```python
from build123d import *
from build123d.topology import SkipClean

# Parameters (mm, degrees)
SKETCH_1_W          = 20
SKETCH_1_H          = 12
SKETCH_1_R          = 2.05
SKETCH_1_R_2        = 3.5
EXTRUDE_1_DEPTH     = 2
CUT_EXTRUDE_START   = 2
SKETCH_1_3_R        = 1.6
CUT_EXTRUDE_6_DEPTH = 1
SKETCH_3_W          = 20
SKETCH_3_H          = 12
EXTRUDE_3_DEPTH     = 1.4
EXTRUDE_START       = 1.4
SKETCH_3_17_W       = 20
SKETCH_3_17_H       = 12
EXTRUDE_4_DEPTH     = 1.7
CUT_EXTRUDE_START_2 = 5.1
SKETCH_5_R          = 0.9
CUT_EXTRUDE_1_DEPTH = 29.974882199
SKETCH_5_10_R       = 1.5
CUT_EXTRUDE_3_DEPTH = 4.6
SKETCH_7_R          = 0.35
SKETCH_7_R_2        = 0.7
CUT_EXTRUDE_4_DEPTH = 24.874882199
SKETCH_7_3_R        = 1
CUT_EXTRUDE_7_DEPTH = 3.1


with BuildPart() as part:
    # 草图1 → 凸台-拉伸1 (new body)
    with BuildSketch(Plane(origin=(0, 0, 0), x_dir=(1, 0, 0), z_dir=(0, 1, 0))):
        with Locations((10, -6)):
            Rectangle(SKETCH_1_W, SKETCH_1_H)
        with Locations(Location((5, -6, 0), (0, 0, 270))):
            Circle(SKETCH_1_R, mode=Mode.SUBTRACT)
        with Locations(Location((15, -6, 0), (0, 0, 270))):
            Circle(SKETCH_1_R_2, mode=Mode.SUBTRACT)
    extrude(amount=EXTRUDE_1_DEPTH)

    # 草图1<3> → 切除-拉伸6 (cut)
    with BuildSketch(Plane(origin=(0, 0, 0), x_dir=(1, 0, 0), z_dir=(0, 1, 0)).offset(CUT_EXTRUDE_START)):
        with Locations(Location((9.2, -6, 0), (0, 0, 270))):
            Circle(SKETCH_1_3_R)
    extrude(amount=-CUT_EXTRUDE_6_DEPTH, mode=Mode.SUBTRACT)

    # 草图3 → 凸台-拉伸3 (add)
    with SkipClean():  # the faces are left unmerged after this step: merging them gives an invalid solid
        with BuildSketch(Plane(origin=(0, 2, 0), x_dir=(1, 0, 0), z_dir=(0, 1, 0))):
            with Locations((10, -6)):
                Rectangle(SKETCH_3_W, SKETCH_3_H)
            with BuildLine():
                ThreePointArc((6.141964286, -7.702473956), (2.95, -6), (6.141964286, -4.297526044))
                ThreePointArc((6.141964286, -4.297526044), (9.04909865, -2.503254544), (12.1, -4.040408206))
                ThreePointArc((12.1, -4.040408206), (18.5, -6), (12.1, -7.959591794))
                ThreePointArc((12.1, -7.959591794), (9.04909865, -9.496745456), (6.141964286, -7.702473956))
            make_face(mode=Mode.SUBTRACT)
        extrude(amount=EXTRUDE_3_DEPTH)

    # 草图3<17> → 凸台-拉伸4 (add)
    with SkipClean():  # the faces are left unmerged after this step: merging them gives an invalid solid
        with BuildSketch(Plane(origin=(0, 2, 0), x_dir=(1, 0, 0), z_dir=(0, 1, 0)).offset(EXTRUDE_START)):
            with Locations((10, -6)):
                Rectangle(SKETCH_3_17_W, SKETCH_3_17_H)
            with BuildLine():
                ThreePointArc((6.141964286, -7.702473956), (2.95, -6), (6.141964286, -4.297526044))
                ThreePointArc((6.141964286, -4.297526044), (8.789071626, -2.524206872), (11.776724138, -3.631352133))
                ThreePointArc((11.776724138, -3.631352133), (16.246374051, -2.199138029), (19, -6))
                ThreePointArc((19, -6), (16.246374051, -9.800861971), (11.776724138, -8.368647867))
                ThreePointArc((11.776724138, -8.368647867), (8.789071626, -9.475793128), (6.141964286, -7.702473956))
            make_face(mode=Mode.SUBTRACT)
        extrude(amount=EXTRUDE_4_DEPTH)

    # 草图5 → 切除-拉伸1 (cut, through all)
    with SkipClean():  # the faces are left unmerged after this step: merging them gives an invalid solid
        with BuildSketch(Plane(origin=(0, 0, 0), x_dir=(1, 0, 0), z_dir=(0, 1, 0)).offset(CUT_EXTRUDE_START_2)):
            with Locations(Location((2.3, -2.214171161, 0), (0, 0, 270))):
                Circle(SKETCH_5_R)
            with Locations(Location((7.7, -9.785828839, 0), (0, 0, 270))):
                Circle(SKETCH_5_R)
        extrude(amount=-CUT_EXTRUDE_1_DEPTH, mode=Mode.SUBTRACT)

    # 草图5<10> → 切除-拉伸3 (cut)
    with SkipClean():  # the faces are left unmerged after this step: merging them gives an invalid solid
        with BuildSketch(Plane(origin=(0, 0, 0), x_dir=(1, 0, 0), z_dir=(0, 1, 0)).offset(CUT_EXTRUDE_START_2)):
            with Locations(Location((2.3, -2.214171161, 0), (0, 0, 270))):
                Circle(SKETCH_5_10_R)
            with Locations(Location((7.7, -9.785828839, 0), (0, 0, 270))):
                Circle(SKETCH_5_10_R)
        extrude(amount=-CUT_EXTRUDE_3_DEPTH, mode=Mode.SUBTRACT)

    # 草图7 → 切除-拉伸4 (cut, through all)
    with SkipClean():  # the faces are left unmerged after this step: merging them gives an invalid solid
        with BuildSketch(Plane(origin=(0, 5.1, 0), x_dir=(1, 0, 0), z_dir=(0, 1, 0))):
            with Locations(Location((6, -2, 0), (0, 0, 270))):
                Circle(SKETCH_7_R)
            with Locations(Location((3, -9, 0), (0, 0, 270))):
                Circle(SKETCH_7_R)
            with Locations(Location((17, -1.5, 0), (0, 0, 270))):
                Circle(SKETCH_7_R)
            with Locations(Location((17, -10.5, 0), (0, 0, 270))):
                Circle(SKETCH_7_R)
            with Locations(Location((11.5, -1.5, 0), (0, 0, 270))):
                Circle(SKETCH_7_R_2)
            with Locations(Location((18.5, -10.5, 0), (0, 0, 270))):
                Circle(SKETCH_7_R_2)
            with Locations(Location((11.5, -10.5, 0), (0, 0, 270))):
                Circle(SKETCH_7_R_2)
            with Locations(Location((18.5, -1.5, 0), (0, 0, 270))):
                Circle(SKETCH_7_R_2)
        extrude(amount=-CUT_EXTRUDE_4_DEPTH, mode=Mode.SUBTRACT)

    # 草图7<3> → 切除-拉伸7 (cut)
    with SkipClean():  # the faces are left unmerged after this step: merging them gives an invalid solid
        with BuildSketch(Plane(origin=(0, 5.1, 0), x_dir=(1, 0, 0), z_dir=(0, 1, 0))):
            with Locations(Location((11.5, -1.5, 0), (0, 0, 270))):
                Circle(SKETCH_7_3_R)
            with Locations(Location((18.5, -10.5, 0), (0, 0, 270))):
                Circle(SKETCH_7_3_R)
            with Locations(Location((11.5, -10.5, 0), (0, 0, 270))):
                Circle(SKETCH_7_3_R)
            with Locations(Location((18.5, -1.5, 0), (0, 0, 270))):
                Circle(SKETCH_7_3_R)
        extrude(amount=-CUT_EXTRUDE_7_DEPTH, mode=Mode.SUBTRACT)


solid = part.part
```
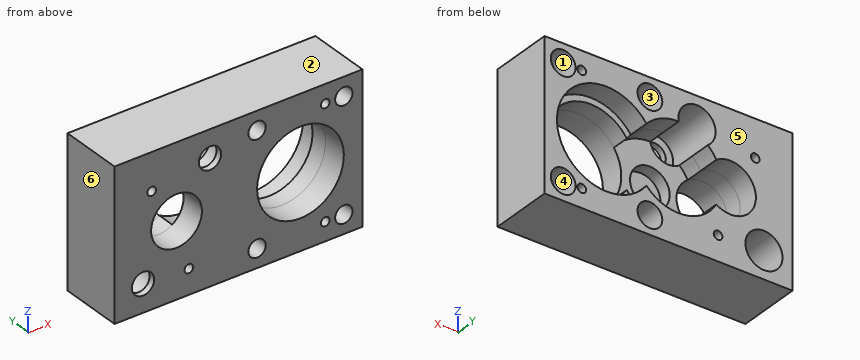
Work out the finished part from the listing and answer in its coordinate system (mm). Face numbers are marked on the shaded views. A direction names the side the tool comes from. Give positions to 0.01 mm unless a question says otherwise; leave off trailing zeros. Order: outer loops, then holes, each group sorted by start corner. A loop starts at its lowest first (then second) coordinate and runs counter-clockwise, first axis right, second up. Notation, with made-up numbers: (-30, -39) - (8, -39) arc R33 cw to (8, -4) - close; hole circle Ø4 at (35, 76.5). An arc over 180 degrees is marked (long way). One line per item, written item: value. Start each with the question number.
1. Section C-C, the plane y = 2.7 is taken. Count the separate pieces of the cut face and the enclosed holes in it, then the cut area to 3 significant figures.
2. Section D-D, the plane x = 5 is taken. Write down the section's boundary in (y, z), then the cut area to 3 significant figures.
3. Consider line 1 (Z direction, x = 2.75, y = 2.2); line 2 (X direction, y = 1.75, z = 5.25); line 3 (X direction, y = 3.05, z = 1.5). Determine where each line is inside the solid, lowest interval first.
4. Section A-A, the plane x = 15 is taken. Write down the section's boundary in (y, z), then the cut area to 3 significant figures.
5. Which of the six approach directions +Z, -Z, +X, -X, +Y, -Y give full straight-line access (tool end or side, diameter ignored) to the marked faces 1 and 2?
6. For a pull along X with two mould halves and no side action, classify the marked faces 3, 4, 5 and 6 as released by +X, released by -X, zero draft, split by the parting line, or undercut.
7. Each of these flat-tipped pins is pushed along its axis until it touches: pin 1 Ø2.5 at (x, z) = (18.5, 10.5) entering from -Y; pin 2 Ø1 at (x, z) = (18.5, 10.5) entering from +Y; pin 3 Ø1 at (x, z) = (9, 5.5) entering from +Y. Where does it stop, or does it pass through?
8. Section B-B, the plane z = 5 is taken. Write down the section's boundary in (x, y), then the cut area to 3 significant figures.
Filled sheet:
1. separate pieces: 1
1. enclosed holes: 10
1. area: 130 mm²
2. outline: (0, 0) - (5.1, 0) - (5.1, 3.95) - (0, 3.95) - close; (0, 8.05) - (5.1, 8.05) - (5.1, 12) - (0, 12) - close
2. area: 40.3 mm²
3. line 1: 0 to 0.78, 3.65 to 8.76, 9.24 to 12
3. line 2: 0 to 3.09, 6.91 to 7.79, 10.61 to 11.58, 18.42 to 20
3. line 3: 0 to 0.98, 3.62 to 10.5, 12.5 to 16.65, 17.35 to 17.5, 19.5 to 20
4. outline: (0, 0) - (5.1, 0) - (5.1, 2) - (3.4, 2) - (3.4, 2.5) - (0, 2.5) - close; (0, 9.5) - (3.4, 9.5) - (3.4, 10) - (5.1, 10) - (5.1, 12) - (0, 12) - close
4. area: 23.8 mm²
5. face 1: +Y
5. face 2: +Z, +X, -X, +Y, -Y
6. face 3: undercut
6. face 4: undercut
6. face 5: zero draft
6. face 6: released by -X
7. pin 1: y = 0
7. pin 2: through
7. pin 3: y = 1
8. outline: (0, 0) - (3.21, 0) - (3.21, 5.1) - (0, 5.1) - close; (6.79, 0) - (11.65, 0) - (11.65, 2) - (10.45, 2) - (10.45, 1) - (7.95, 1) - (7.95, 2) - (6.79, 2) - close; (18.35, 0) - (20, 0) - (20, 5.1) - (18.87, 5.1) - (18.87, 3.4) - (18.35, 3.4) - close
8. area: 31.1 mm²
